from build123d import *

# Parameters (mm, degrees)
SKETCH1_9_W                                = 170
SKETCH1_9_H                                = 87
BOSS_EXTRUDE5_DEPTH                        = 2
SKETCH1_10_W                               = 63
SKETCH1_10_H                               = 78
CUT_EXTRUDE3_DEPTH                         = 9
SKETCH1_12_W                               = 170
SKETCH1_12_H                               = 87
BOSS_EXTRUDE6_DEPTH                        = 14
SKETCH1_W                                  = 63
SKETCH1_H                                  = 78
CUT_EXTRUDE4_DEPTH                         = 29
SKETCH8_W                                  = 83.526029731
SKETCH8_H                                  = 10.5
CUT_EXTRUDE5_DEPTH                         = 168
BOSS_EXTRUDE10_DEPTH                       = 22.5
CHAMFER1_SIZE                              = 10
CHAMFER2_SIZE                              = 10
SKETCH47_R                                 = 2.15
CUT_EXTRUDE10_DEPTH                        = 9.5
SKETCH37_W                                 = 170
SKETCH37_H                                 = 9
BOSS_EXTRUDE20_DEPTH                       = 5
SKETCH25_W                                 = 170
SKETCH25_H                                 = 8
BOSS_EXTRUDE18_DEPTH                       = 120
SKETCH28_W                                 = 170
SKETCH28_H                                 = 8
BOSS_EXTRUDE19_DEPTH                       = 120
SKETCH43_W                                 = 146
SKETCH43_H                                 = 110
CUT_EXTRUDE9_DEPTH                         = 170.5
SKETCH42_W                                 = 63
SKETCH42_H                                 = 3.5
BOSS_EXTRUDE22_DEPTH                       = 20.5
SKETCH38_W                                 = 5
SKETCH38_H                                 = 9
BOSS_EXTRUDE23_DEPTH                       = 9.5
MIRROR14_AT_THE_SECOND_PLANE_COPY_1_SKET_W = 5
MIRROR14_AT_THE_SECOND_PLANE_COPY_1_SKET_H = 9
MIRROR14_AT_THE_SECOND_PLANE_COPY_1_DEPTH  = 9.5


with BuildPart() as part:
    # Sketch1<9> → Boss-Extrude5 (new body)
    with BuildSketch(Plane(origin=(0, 0, 0), x_dir=(1, 0, 0), z_dir=(0, 1, 0))):
        with Locations((82.5, 41)):
            Rectangle(SKETCH1_9_W, SKETCH1_9_H)
    extrude(amount=BOSS_EXTRUDE5_DEPTH)

    # Sketch1<10> → Cut-Extrude3 (cut)
    with BuildSketch(Plane(origin=(0, 0, 0), x_dir=(1, 0, 0), z_dir=(0, 1, 0))):
        with Locations((131.5, 41)):
            Rectangle(SKETCH1_10_W, SKETCH1_10_H)
    extrude(amount=CUT_EXTRUDE3_DEPTH, mode=Mode.SUBTRACT)

    # Sketch1<12> → Boss-Extrude6 (add)
    with BuildSketch(Plane(origin=(0, 0, 0), x_dir=(1, 0, 0), z_dir=(0, 1, 0))):
        with Locations((82.5, 41)):
            Rectangle(SKETCH1_12_W, SKETCH1_12_H)
    extrude(amount=BOSS_EXTRUDE6_DEPTH)

    # Sketch1 → Cut-Extrude4 (cut)
    with BuildSketch(Plane(origin=(0, 0, 0), x_dir=(1, 0, 0), z_dir=(0, 1, 0))):
        with Locations((131.5, 41)):
            Rectangle(SKETCH1_W, SKETCH1_H)
    extrude(amount=CUT_EXTRUDE4_DEPTH, mode=Mode.SUBTRACT)

    # Sketch8 → Cut-Extrude5 (cut)
    with BuildSketch(Plane.ZY.offset(2.5)):
        with Locations((-40.910699185, 8.75)):
            Rectangle(SKETCH8_W, SKETCH8_H)
    extrude(amount=-CUT_EXTRUDE5_DEPTH, mode=Mode.SUBTRACT)

    # Sketch11 → Boss-Extrude10 (add)
    with BuildSketch(Plane.XY.offset(2.5)):
        Polygon((-2.5, 14), (90, 14), (167.5, 14), (167.5, 9), (90, 9), (-2.5, 9), align=None)
    boss_extrude10 = extrude(amount=BOSS_EXTRUDE10_DEPTH)

    # Mirror10: Boss-Extrude10 across plane
    add(boss_extrude10.mirror(Plane.XY.offset(-41)))

    # Chamfer1
    # the kernel refuses this chamfer: 10 mm, written as the material it adds along each edge
    with BuildSketch(Plane(origin=(-2.5, 9, 2.5), x_dir=(0, -0.9996219169112968, -0.02749587661058636), z_dir=(1, 0, 0))) as chamfer1_piece_1_section:
        Polygon((CHAMFER1_SIZE * 0.999621916911, -CHAMFER1_SIZE * 0.0274958766106), (-CHAMFER1_SIZE * 0.0274958766106, -CHAMFER1_SIZE * 0.999621916911), (0, 0), align=None)
    chamfer1_piece_1 = extrude(amount=170, mode=Mode.PRIVATE)
    chamfer1_piece_1 = split(chamfer1_piece_1, bisect_by=Plane(origin=(82.5, 0, 5.859007471), z_dir=(0, 1, 0)), keep=Keep.TOP, mode=Mode.PRIVATE)
    add(chamfer1_piece_1)

    # Chamfer2
    # the kernel refuses this chamfer: 10 mm, written as the material it adds along each edge
    with BuildSketch(Plane(origin=(-2.5, 9, -84.5), x_dir=(0, 0.027495876610586317, -0.9996219169112968), z_dir=(1, 0, 0))) as chamfer2_piece_1_section:
        Polygon((CHAMFER2_SIZE * 0.999621916911, -CHAMFER2_SIZE * 0.0274958766106), (-CHAMFER2_SIZE * 0.0274958766106, -CHAMFER2_SIZE * 0.999621916911), (0, 0), align=None)
    chamfer2_piece_1 = extrude(amount=170, mode=Mode.PRIVATE)
    chamfer2_piece_1 = split(chamfer2_piece_1, bisect_by=Plane(origin=(82.5, 0, -87.859007471), z_dir=(0, 1, 0)), keep=Keep.TOP, mode=Mode.PRIVATE)
    add(chamfer2_piece_1)

    # Sketch47 → Cut-Extrude10 (cut)
    with BuildSketch(Plane(origin=(0, 14, 0), x_dir=(1, 0, 0), z_dir=(0, 1, 0))):
        with Locations(Location((5.5, 100, 0), (0, 0, 270))):
            Circle(SKETCH47_R)
        with Locations(Location((159.5, 100, 0), (0, 0, 270))):
            Circle(SKETCH47_R)
        with Locations(Location((159.5, -18, 0), (0, 0, 90))):
            Circle(SKETCH47_R)
        with Locations(Location((5.5, -18, 0), (0, 0, 90))):
            Circle(SKETCH47_R)
    extrude(amount=-CUT_EXTRUDE10_DEPTH, mode=Mode.SUBTRACT)

    # Sketch37 → Boss-Extrude20 (add)
    with BuildSketch(Plane.XY.offset(2.5)):
        with Locations((82.5, 4.5)):
            Rectangle(SKETCH37_W, SKETCH37_H)
    boss_extrude20 = extrude(amount=BOSS_EXTRUDE20_DEPTH)

    # Sketch25 → Boss-Extrude18 (add)
    with BuildSketch(Plane.XZ.offset(-9)):
        with Locations((82.5, -103)):
            Rectangle(SKETCH25_W, SKETCH25_H)
    extrude(amount=BOSS_EXTRUDE18_DEPTH)

    # Sketch28 → Boss-Extrude19 (add)
    with BuildSketch(Plane.XZ.offset(-9)):
        with Locations((82.5, 21)):
            Rectangle(SKETCH28_W, SKETCH28_H)
    extrude(amount=BOSS_EXTRUDE19_DEPTH)

    # Mirror11: Boss-Extrude20 across plane
    add(boss_extrude20.mirror(Plane.XY.offset(-41)))

    # Sketch43 → Cut-Extrude9 (cut)
    with BuildSketch(Plane.XY.offset(25)):
        with Locations((82.5, -56)):
            Rectangle(SKETCH43_W, SKETCH43_H)
    extrude(amount=-CUT_EXTRUDE9_DEPTH, mode=Mode.SUBTRACT)

    # Sketch42 → Boss-Extrude22 (add)
    with BuildSketch(Plane(origin=(0, 0, -2), x_dir=(-1, 0, 0), z_dir=(0, 0, -1))):
        with Locations((-131.5, 1.75)):
            Rectangle(SKETCH42_W, SKETCH42_H)
    extrude(amount=BOSS_EXTRUDE22_DEPTH)

    # Sketch38 → Boss-Extrude23 (add)
    with BuildSketch(Plane.XY.offset(7.5)):
        with Locations((0, 4.5)):
            Rectangle(SKETCH38_W, SKETCH38_H)
    boss_extrude23 = extrude(amount=BOSS_EXTRUDE23_DEPTH)

    # Mirror14: Boss-Extrude23 across plane
    add(boss_extrude23.mirror(Plane.XY.offset(-41)))

    # Mirror14 at the second plane: Boss-Extrude23 across plane
    add(boss_extrude23.mirror(Plane.ZY.offset(-82.5)))

    # Mirror14 at the second plane copy 1 sket → Mirror14 at the second plane copy 1 (add)
    with BuildSketch(Plane(origin=(165, 0, -89.5), x_dir=(-1, 0, 0), z_dir=(0, 0, -1))):
        with Locations((0, 4.5)):
            Rectangle(MIRROR14_AT_THE_SECOND_PLANE_COPY_1_SKET_W, MIRROR14_AT_THE_SECOND_PLANE_COPY_1_SKET_H)
    extrude(amount=MIRROR14_AT_THE_SECOND_PLANE_COPY_1_DEPTH)


solid = part.part
Model file for the job. Use its own axes, mm. A direction names the side the tool comes from. Give positions to 0.01 mm unless a question says otherwise; leave off trailing zeros. Loops run counter-clockwise (first coordinate to the right, second up) from the corner with the lowest first, then second, coordinate; pieces in that order, holes last.
Item 1: Slice it at C-C (x = 134). Write the cut outline in (y, z), plus the area to 3 significant figures.
Check values:
outline: (-1, -107) - (14, -107) - (14, -82.67) - (3.5, -82.67) - (3.5, -80) - (0, -80) - (0, -89.5) - (4, -89.5) - (9, -94.5) - (9, -99) - (-1, -99) - close; (-1, 17) - (9, 17) - (9, 12.5) - (4, 7.5) - (0, 7.5) - (0, -22.5) - (3.5, -22.5) - (3.5, 0.85) - (14, 0.85) - (14, 25) - (-1, 25) - close
area: 640 mm2
Item 2: Slice it at A-A (z = -44.5). Write the cut outline in (x, y), plus the area to 4 significant figures.
Check values:
outline: (-2.5, 0) - (100, 0) - (100, 3.5) - (-2.5, 3.5) - close; (163, 0) - (167.5, 0) - (167.5, 14) - (165.5, 14) - (165.5, 3.5) - (163, 3.5) - close
area: 395.5 mm2
Item 3: Drill centre lines: line 1 along Z through (x, y) = (113, 1.5); line 2 along X through (y, z) = (10, -100); line 3 along Z through (x, y) = (159.5, 10.7). Where is each one in solid material? Low to high.
Check values:
line 1: z = -107 to -99, -89.5 to -80, -22.5 to 7.5, 17 to 25
line 2: x = -2.5 to 3.35, 7.65 to 157.35, 161.65 to 167.5
line 3: z = -107 to -102.15, -97.85 to -82.67, 0.85 to 15.85, 20.15 to 25
Item 4: Drop flat-ended pins along their axis: P1, Ø5, axis at x = 34, z = -80, coming from the -Y side; P2, Ø0.9, axis at x = 159, z = -100, coming from the +Y side; P3, Ø2.5, axis at x = 94, z = 19.5, coming from the -Y side. Give the stop position or say it passes through.
Check values:
P1: stops at y = 0
P2: stops at y = 9
P3: stops at y = -1
Item 5: Which spindle directions (+Z, -Z, +X, -X, +Y, -Y) get a long thin tool onto all of the face, cutting with end or side? Do faces 1 (the face through (161.6, 11.54, 18.47)), 2 (the face through (155.5, -57, 21)), 3 (the face through (65, 0, -40)), 4 (the face through (81, 9, 15)). Say none if no direction does.
Check values:
face 1: +Y
face 2: +Z, -Z, -Y
face 3: +X, -X, -Y
face 4: -Y
Item 6: Slice it at D-D (x = 64). Write the cut outline in (y, z).
Check values:
outline: (-1, -107) - (14, -107) - (14, -82.67) - (3.5, -82.67) - (3.5, 0.85) - (14, 0.85) - (14, 25) - (-1, 25) - (-1, 17) - (9, 17) - (9, 12.5) - (4, 7.5) - (0, 7.5) - (0, -89.5) - (4, -89.5) - (9, -94.5) - (9, -99) - (-1, -99) - close
Item 7: Mould opens along Z. For faces 5 (the face through (81, 9, -97)), 6 (the face through (167.5, 2, -36)), 7 (the face through (162.5, 4, 12)) say: +Z half, -Z half, draft (parallel to the pull), parting line (faces both ways), or undercut.
Check values:
face 5: undercut
face 6: draft
face 7: undercut
Item 8: Slice it at B-B (y = -43.5). Write the cut outline in (x, z), plus the area to 3 significant figures.
Check values:
outline: (-2.5, -107) - (9.5, -107) - (9.5, -99) - (-2.5, -99) - close; (-2.5, 17) - (9.5, 17) - (9.5, 25) - (-2.5, 25) - close; (155.5, -107) - (167.5, -107) - (167.5, -99) - (155.5, -99) - close; (155.5, 17) - (167.5, 17) - (167.5, 25) - (155.5, 25) - close
area: 384 mm2
